from build123d import *

# Parameters (mm, degrees)
BOSS_EXTRUDE2_DEPTH = 6.35
SKETCH3_R           = 6.35
CUT_EXTRUDE1_DEPTH  = 6.35


with BuildPart() as part:
    # Sketch2 → Boss-Extrude2 (new body)
    with BuildSketch(Plane(origin=(0, 0, 0), x_dir=(1, 0, 0), z_dir=(0, 1, 0))):
        with BuildLine():
            Line((0, 0), (0, 38.1))
            ThreePointArc((0, 38.1), (-26.940768363, 26.940768363), (-38.1, 0))
            Line((-38.1, 0), (0, 0))
        make_face()
        with BuildLine():
            Line((19.05, 0), (38.1, 0))
            ThreePointArc((38.1, 0), (26.940768363, 26.940768363), (0, 38.1))
            Line((0, 38.1), (0, 0))
            Line((0, 0), (19.05, 0))
        make_face()
        with BuildLine():
            Line((19.05, -19.05), (19.05, 0))
            Line((19.05, 0), (38.1, 0))
            ThreePointArc((38.1, 0), (32.520384182, -13.470384182), (19.05, -19.05))
        make_face()
        with BuildLine():
            Line((0, 0), (19.05, 0))
            Line((19.05, 0), (19.05, -19.05))
            ThreePointArc((19.05, -19.05), (5.579615818, -13.470384182), (0, 0))
        make_face()
    extrude(amount=BOSS_EXTRUDE2_DEPTH)

    # Sketch3 → Cut-Extrude1 (cut)
    with BuildSketch(Plane(origin=(0, 6.35, 0), x_dir=(1, 0, 0), z_dir=(0, 1, 0))):
        with Locations(Location((19.05, 0, 0), (0, 0, 270))):
            Circle(SKETCH3_R)
    extrude(amount=-CUT_EXTRUDE1_DEPTH, mode=Mode.SUBTRACT)


solid = part.part
Source: CAD feature listing. Evaluate the final solid. Frame: model axes, mm. A direction names the side the tool comes from. Give positions to 0.01 mm unless a question says otherwise; leave off trailing zeros. Loops run counter-clockwise (first coordinate to the right, second up) from the corner with the lowest first, then second, coordinate; pieces in that order, holes last. Notation, with made-up numbers: (37, -15.75) -> (89, -15.75) arc R21 ccw to (89, 4.25) -> close; hole circle Ø11 at (46, 46). An arc over 180 degrees is marked (long way). Use a Markdown table: item, result. Add a question column.
1) Reachability of faces 1 (the face through (-1, 0, -10)), 2 (the face through (-19, 3, 0)) from +Z, -Z, +X, -X, +Y, -Y: full face, straight path, thin tool, end or side. Return the list, or none.
2) Line query: line 1 along Z through (x, y) = (17.5, 3.25); line 2 along X through (y, z) = (1, -22.5); line 3 along Z through (x, y) = (-30, 2.5). Output: solid intervals per line, ascending. Write a range as [from, to].
3) Section query B-B, the plane z = -2. Return the cut outline in (x, y), then the cut area to 3 significant figures.
4) Section query C-C, the plane z = 4. Return the cut outline in (x, y).
5) First-contact query: pin 1 (2 mm diameter, centred on x = -29, y = 4.5, fed in from +Z). Flat tip, straight axial feed; report the tip coordinate or a pass-through.
6) Section query D-D, the plane z = -16. Return the cut outline in (x, y).
7) Section query A-A, the plane y = 2.25. Return the cut outline in (x, z), then the cut area to 3 significant figures.
8) Pull-direction query (X, two-part tool) for faces 3 (the face through (25.346, 3.219, -0.827)), 4 (the face through (-1, 6.35, -10)); classes: +X half, -X half, draft (parallel to the pull), parting line (faces both ways), or undercut.
Numbers:
| question | item | result |
|---|---|---|
| 1 | face 1 | +Z, -Z, +X, -X, -Y |
| 1 | face 2 | +Z, -X, +Y, -Y |
| 2 | line 1 | z = [-33.84, -6.16], [6.16, 18.99] |
| 2 | line 2 | x = [-30.75, 30.75] |
| 2 | line 3 | z = [-23.49, 0] |
| 3 | outline | (-38.05, 0) -> (13.02, 0) -> (13.02, 6.35) -> (-38.05, 6.35) -> close; (25.08, 0) -> (38.05, 0) -> (38.05, 6.35) -> (25.08, 6.35) -> close |
| 3 | area | 407 mm2 |
| 4 | outline | (0.42, 0) -> (14.12, 0) -> (14.12, 6.35) -> (0.42, 6.35) -> close; (23.98, 0) -> (37.68, 0) -> (37.68, 6.35) -> (23.98, 6.35) -> close |
| 5 | pin 1 | stops at z = 0 |
| 6 | outline | (-34.58, 0) -> (34.58, 0) -> (34.58, 6.35) -> (-34.58, 6.35) -> close |
| 7 | outline | (-38.1, 0) arc R38.1 ccw to (38.1, 0) arc R19.05 ccw to (0, 0) -> close; hole circle Ø12.7 at (19.05, 0) |
| 7 | area | 2,720 mm2 |
| 8 | face 3 | undercut |
| 8 | face 4 | draft |
